Work out the finished part from the listing and answer in its coordinate system (mm). Face numbers are marked on the shaded views. A direction names the side the tool comes from. Round coordinates to 2 decimals unless told otherwise and drop trailing zeros. Loops run counter-clockwise (first coordinate to the right, second up) from the corner with the lowest first, then second, coordinate; pieces in that order, holes last.
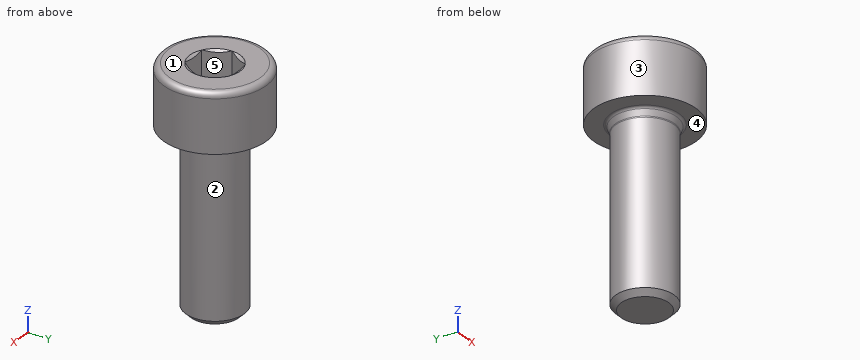
Solid Edge part; units mm, degrees
sketch "Sketch1" plane through (0, 0, 0) normal (0, 0, 1) x (1, 0, 0)
  line L0 (-0.866, 1.5) -> (0.866, 1.5)
  line L1 (0.866, 1.5) -> (1.7321, 0)
  line L2 (1.7321, 0) -> (0.866, -1.5)
  line L3 (0.866, -1.5) -> (-0.866, -1.5)
  line L4 (-0.866, -1.5) -> (-1.7321, 0)
  line L5 (-1.7321, 0) -> (-0.866, 1.5)
  circle A0 centre (0, 0) radius 3.5
extrude "Protrusion1" add sketch "Sketch1" along normal blind 4
sketch "Sketch2" plane through (0, 0, 0) normal (0, -1, 0) x (1, 0, 0)
  line L0 (0, 1) -> (1.7321, 2)
  line L1 (1.7321, 2) -> (3.5, 2)
  line L2 (3.5, 2) -> (3.5, 0)
  line L3 (3.5, 0) -> (2, 0)
  line L4 (2, 0) -> (2, -0.6)
  line L5 (2, -0.6) -> (2, -0.601) construction
  line L6 (2, -0.601) -> (2, -0.601) construction
  line L7 (2, -0.601) -> (2, -12)
  line L8 (0, -12) -> (2, -12)
revolve "RevolvedProtrusion_1" add sketch "Sketch2" angle 360 about axis through (0, 0, 2.3333) along (0, 0, -1)
cosmetic_thread "Thread_1" thread depth 11.398
sketch "Sketch3" plane through (0, 0, 0) normal (0, -1, 0) x (1, 0, 0)
  line L0 (0, 5) -> (1.72, 5)
  line L1 (1.72, 5) -> (1.72, 4)
  line L2 (1.72, 4) -> (0, 3.007)
revolve "RevolvedCutout_1" cut sketch "Sketch3" angle 360 about axis through (0, 0, 7.1999) along (0, 0, 1)
fillet "Round_1" radius 0.4 1 edges at (-3.5, 0, 4)
sketch "Sketch4" plane through (0, 0, 0) normal (0, -1, 0) x (1, 0, 0)
  line L0 (2, 0) -> (2.35, 0)
  arc A0 (2.1627, -0.1298) -> (2.35, 0) centre (2.35, -0.2) cw
  line L1 (2.0127, -0.5298) -> (2.1627, -0.1298)
  arc A1 (2.0127, -0.5298) -> (2, -0.6) centre (2.2, -0.6) ccw
  line L2 (2, 0) -> (2, -0.6)
revolve "RevolvedProtrusion_2" add sketch "Sketch4" angle 360 about axis through (0, 0, -1.02) along (0, 0, 1)
chamfer "Chamfer_1" distance 0.379 angle 45 1 edges at (-2, 0, -12)
properties material "Acier"
Item 1: For the marked faces 1 and 2, determine the directions among +Z, -Z, +X, -X, +Y, -Y from which every point of the face is accessible in a straight line to the end or side of a thin tool.
Item 2: Determine the mould class of the marked faces 3, 4 and 5 for opening direction Y: pulls with the +Y half, pulls with the -Y half, needs draft (parallel to the pull), parting line crosses it, or undercut.
Item 3: Each of these flat-tipped pins is pushed along its axis until it touches: P1, Ø4, axis at x = 2.5, z = 2, coming from the -Y side; P2, Ø3, axis at y = 2.5, z = -5, coming from the -X side; P3, Ø1.5, axis at x = -2, z = 1.5, coming from the +Y side. Where does it stop, or does it pass through?
Item 4: Section A-A, the plane z = -2.75 is taken. Give the vertices of the cut face in (x, y), plus the area to 3 significant figures.
Item 5: Straight lines are drawn through the part: line 1 (X direction, y = 2.75, z = 2.75); line 2 (Z direction, x = -2.25, y = -1). For each, find the intervals that lie inside material, in ascending order.
Answer below:
1. face 1: +Z, +X, -X, +Y, -Y
1. face 2: -Z
2. face 3: parting line crosses it
2. face 4: needs draft
2. face 5: undercut
3. P1: stops at y = -3.46
3. P2: stops at x = -1.73
3. P3: stops at y = 3.27
4. outline: circle Ø4 at (0, 0)
4. area: 12.6 mm2
5. line 1: x = -2.17 to 2.17
5. line 2: z = 0 to 4
